Design review of the part built by this model. Coordinates are the model's own, in mm. Give positions to 0.01 mm unless a question says otherwise; leave off trailing zeros. Write each loop counter-clockwise with the first axis right and the second up, starting at its lowest first coordinate (ties: lowest second). Pieces come first, ordered by that corner, then holes. Notation, with made-up numbers: (70, -1) -> (129, -1) arc R14 cw to (129, 16) -> close; hole circle Ø4 at (-4.75, 11.25). An arc over 180 degrees is marked (long way). Use CSV: the item, a comma, the result in double quotes.
```python
from build123d import *

# Parameters (mm, degrees)
SALIENTE_EXTRUIR1_DEPTH = 4
REDONDEO1_R             = 1
REDONDEO2_R             = 0.5


with BuildPart() as part:
    # Croquis1 → Saliente-Extruir1 (new body)
    with BuildSketch(Plane(origin=(0, 0, 0), x_dir=(1, 0, 0), z_dir=(0, 1, 0))):
        Polygon((3.5, 0), (5.5, 0), (5.5, -15), (0, -15), (0, 0), (2, 0), (2, -13), (3.5, -13), align=None)
    extrude(amount=SALIENTE_EXTRUIR1_DEPTH)

    # Redondeo1
    redondeo1_edges = [part.edges().sort_by_distance(p)[0] for p in [
        (0, 2, 0),
        (5.5, 2, 0),
        (5.5, 2, 15),
        (0, 2, 15),
    ]]
    fillet(redondeo1_edges, radius=REDONDEO1_R)

    # Redondeo2
    redondeo2_edges = [part.edges().sort_by_distance(p)[0] for p in [
        (2, 2, 13),
        (3.5, 2, 13),
    ]]
    fillet(redondeo2_edges, radius=REDONDEO2_R)


solid = part.part
```
(1) Take a section at B-B (y = 2.9). Write out the cut boundary in (x, z), then the cut area to 3 significant figures.
Established:
outline,"(0, 1) arc R1 ccw to (1, 0) -> (2, 0) -> (2, 12.5) arc R0.5 cw to (2.5, 13) -> (3, 13) arc R0.5 cw to (3.5, 12.5) -> (3.5, 0) -> (4.5, 0) arc R1 ccw to (5.5, 1) -> (5.5, 14) arc R1 ccw to (4.5, 15) -> (1, 15) arc R1 ccw to (0, 14) -> close"
area,"62.2 mm2"
(2) For line 1 along X through (y, z) = (0.9, 10); line 2 along Z through (x, y) = (2.95, 0.75), list the stretches that pass through material, from the lowest coordinate up. Write a range as [from, to].
Established:
line 1,"x = [0, 2], [3.5, 5.5]"
line 2,"z = [13, 15]"
(3) Mouldability with a two-part tool opening along X and no side actions: class faces 1 (the face through (4, 2, 0)), 2 (the face through (5.199, 2.028, 0.285)), 3 (the face through (3.5, 2, 6)), 4 (the face through (2, 2, 6)) as +X half, -X half, draft (parallel to the pull), parting line (faces both ways), or undercut.
Established:
face 1,"draft"
face 2,"+X half"
face 3,"undercut"
face 4,"undercut"
(4) Take a section at D-D (x = 0.4). Write out the cut boundary in (y, z).
Established:
outline,"(0, 0.2) -> (4, 0.2) -> (4, 14.8) -> (0, 14.8) -> close"
(5) Take a section at A-A (z = 4). Write out the cut boundary in (x, y), then the cut area to 3 significant figures.
Established:
outline,"(0, 0) -> (2, 0) -> (2, 4) -> (0, 4) -> close; (3.5, 0) -> (5.5, 0) -> (5.5, 4) -> (3.5, 4) -> close"
area,"16.0 mm2"
(6) Take a section at C-C (x = 2.65). Write out the cut boundary in (y, z), then the cut area to 3 significant figures.
Established:
outline,"(0, 13) -> (4, 13) -> (4, 15) -> (0, 15) -> close"
area,"8.00 mm2"
